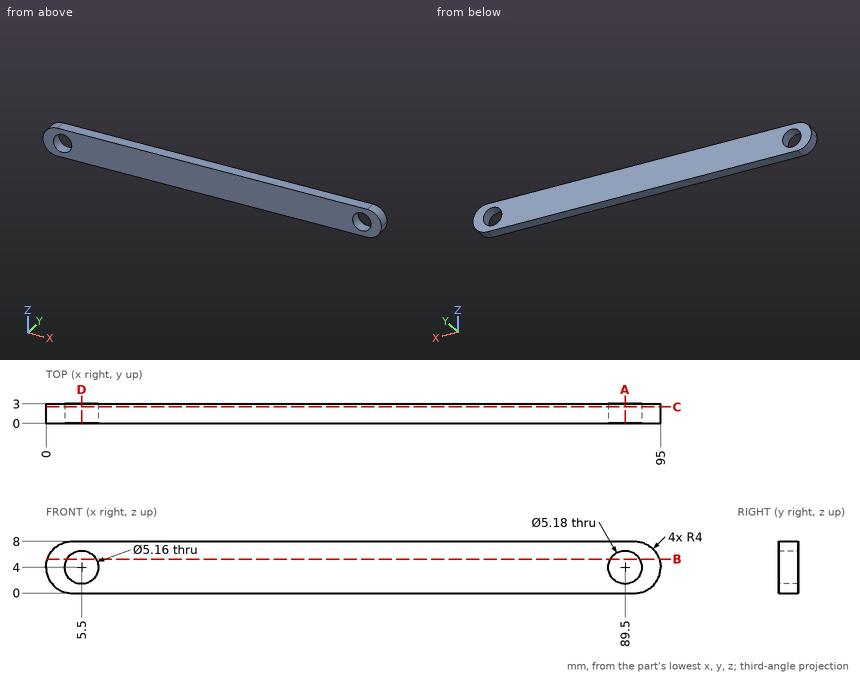
Print and shaded views of the part. All mm, measured from the part's lowest x, y and z. Coordinates: 2 decimals unless noted, no trailing zeros. Order: outer loops, then holes, each group sorted by start corner. A loop starts at its lowest first (then second) coordinate and runs counter-clockwise, first axis right, second up.
Item 1: Drop a flat-ended pin along its axis: pin 1 Ø1 at (y, z) = (1, 7) entering from +X. Give the stop position or say it passes through.
Filled in:
pin 1: stops at x = 94.12
Item 2: Saw through at C-C on y = 2.55. State how many separate pieces and enclosed holes the cut face has, then the cut area to 3 significant figures.
Filled in:
separate pieces: 1
enclosed holes: 2
area: 704 mm2
Item 3: Saw through at A-A on x = 89.5. List the corners of the cut face in (y, z).
Filled in:
outline: (0, 0) - (3, 0) - (3, 1.41) - (0, 1.41) - close; (0, 6.59) - (3, 6.59) - (3, 8) - (0, 8) - close
Item 4: Drill centre lines: L1, parallel to X at y = 2, z = 4; L2, parallel to Z at x = 89.5, y = 1.5; L3, parallel to X at y = 0.2, z = 2.5. Where is each one in solid material? Low to high.
Filled in:
L1: x = 0 to 2.92, 8.08 to 86.91, 92.09 to 95
L2: z = 0 to 1.41, 6.59 to 8
L3: x = 0.29 to 3.4, 7.6 to 87.39, 91.61 to 94.71
Item 5: Saw through at D-D on x = 5.5. List the corners of the cut face in (y, z), then the cut area to 3 significant figures.
Filled in:
outline: (0, 0) - (3, 0) - (3, 1.42) - (0, 1.42) - close; (0, 6.58) - (3, 6.58) - (3, 8) - (0, 8) - close
area: 8.52 mm2
Item 6: Saw through at B-B on z = 5.25. List the corners of the cut face in (x, y), then the cut area to 3 significant figures.
Filled in:
outline: (0.2, 0) - (3.24, 0) - (3.24, 3) - (0.2, 3) - close; (7.76, 0) - (87.23, 0) - (87.23, 3) - (7.76, 3) - close; (91.77, 0) - (94.8, 0) - (94.8, 3) - (91.77, 3) - close
area: 257 mm2
